Check sheet for the modelled part. Datum: model origin and axes. Units: mm. A direction names the side the tool comes from. Round coordinates to 2 decimals unless told otherwise and drop trailing zeros. Order: outer loops, then holes, each group sorted by start corner. A loop starts at its lowest first (then second) coordinate and runs counter-clockwise, first axis right, second up. Notation, with made-up numbers: M -6.75,-29 L 42.25,-29 A26 ccw 42.25,-1 Z; hole C 74.25,-13.75 d2. An arc over 180 degrees is marked long. One line per item, written item: value. Start each with the question number.
(1) Depth check by flat-ended pin: pin 1 Ø1 at (y, z) = (5.5, 10) entering from +X; pin 2 Ø1.5 at (y, z) = (6, 12) entering from -X; pin 3 Ø4 at (y, z) = (7, -7.5) entering from +X. Enter the tip coordinate at first touch or a pass-through.
(2) Access from +Z, -Z, +X, -X, +Y, -Y to the whole of each face (thin tool, end or side, straight path). Record for faces 1 (the face through (90, 5, 17.272)), 2 (the face through (-16, 5, 0)).
(3) Cross-section at A-A, the plane x = 376.5. Enter the section's corners in (y, z).
(4) Cross-section at B-B, the plane z = -9. Enter the section's corners in (x, y), and give its area (3 significant figures).
(5) Release check for a two-part mould opening along X. For faces 3 (the face through (381, 5, 15.748)), 4 (the face through (381, 5, 17.272)), 5 (the face through (532.126, 4.758, -0.606)), 6 (the face through (-17.52, 4.76, 0.13)) record: released by +X, released by -X, zero draft, split by the parting line, or undercut.
(6) Thickness scan on L1, parallel to Z at x = 47, y = 2.75; L2, parallel to X at y = 6.5, z = 1; L3, parallel to Z at x = 217.5, y = 2.5. Record the ranges inside material, lowest first.
from build123d import *

# Parameters (mm, degrees)
BOSS_EXTRUDE1_DEPTH = 9.652
SKETCH2_W           = 63.5
SKETCH2_H           = 9.652
CUT_EXTRUDE1_DEPTH  = 12.7


with BuildPart() as part:
    # Sketch1 → Boss-Extrude1 (new body)
    with BuildSketch(Plane(origin=(0, 0, 0), x_dir=(1, 0, 0), z_dir=(0, 1, 0))):
        with BuildLine():
            Line((0, 17.78), (516.128, 17.78))
            ThreePointArc((516.128, 17.78), (533.654, 0.254), (516.128, -17.272))
            Line((516.128, -17.272), (0, -17.272))
            ThreePointArc((0, -17.272), (-17.526, 0.254), (0, 17.78))
        make_face()
        with BuildLine():
            Line((0, 16.256), (516.128, 16.256))
            ThreePointArc((516.128, 16.256), (532.13, 0.254), (516.128, -15.748))
            Line((516.128, -15.748), (0, -15.748))
            ThreePointArc((0, -15.748), (-16.002, 0.254), (0, 16.256))
        make_face(mode=Mode.SUBTRACT)
    extrude(amount=BOSS_EXTRUDE1_DEPTH)

    # Sketch2 → Cut-Extrude1 (cut)
    with BuildSketch(Plane.XY.offset(17.272)):
        with Locations((209.55, 4.826)):
            Rectangle(SKETCH2_W, SKETCH2_H)
    extrude(amount=-CUT_EXTRUDE1_DEPTH, mode=Mode.SUBTRACT)


solid = part.part
Values found:
1. pin 1: x = 530.69
1. pin 2: x = -13.22
1. pin 3: x = 532.85
2. face 1: +Z, +X, -X, +Y, -Y
2. face 2: +Y, -Y
3. outline: M 0,-17.78 L 9.65,-17.78 L 9.65,-16.26 L 0,-16.26 Z; M 0,15.75 L 9.65,15.75 L 9.65,17.27 L 0,17.27 Z
4. outline: M -15.19,0 L -13.4,0 L -13.4,9.65 L -15.19,9.65 Z; M 529.53,0 L 531.32,0 L 531.32,9.65 L 529.53,9.65 Z
4. area: 34.5 mm^2
5. face 3: undercut
5. face 4: zero draft
5. face 5: undercut
5. face 6: released by -X
6. L1: -17.78 to -16.26, 15.75 to 17.27
6. L2: -17.48 to -15.95, 532.08 to 533.61
6. L3: -17.78 to -16.26
